Model file for the job. Use its own axes, mm. Face numbers are marked on the shaded views. Round coordinates to 2 decimals unless told otherwise and drop trailing zeros. Order: outer loops, then holes, each group sorted by start corner. A loop starts at its lowest first (then second) coordinate and runs counter-clockwise, first axis right, second up. Notation, with made-up numbers: (31.5, -3.75) - (68.5, -3.75) arc R17 ccw to (68.5, 12.25) - close; hole circle Ø2 at (-17, -30.5). An arc over 180 degrees is marked (long way). Put each result on its own line as item: value. Start each with the question number.
Item 1: Mould opens along X. For the marked faces 1, 2, 3 and 4 say: pulls with the +X half, pulls with the -X half, needs draft (parallel to the pull), parting line crosses it, or undercut.
Item 2: Saw through at A-A on x = 0. List the corners of the cut face in (y, z), plus the area to 3 significant figures.
Item 3: Pin check, flat tips, straight feed: pin 1 Ø1.5 at (x, y) = (6.5, 1.5) entering from +Z; pin 2 Ø3 at (x, y) = (7, 1) entering from -Z; pin 3 Ø1.5 at (x, y) = (3.5, 4) entering from -Z. Stop position of each tip, or through.
Item 4: Saw through at C-C on y = 3.4. List the corners of the cut face in (x, z), plus the area to 3 significant figures.
Item 5: Saw through at D-D on z = 9.25. List the corners of the cut face in (x, y), plus the area to 3 significant figures.
Item 6: Saw through at B-B on z = 0. List the corners of the cut face in (x, y), plus the area to 3 significant figures.
Item 7: Probe probe 1 along X at (y, z) = (1.6, 0); probe 2 along Z at (x, y) = (-1.5, 2.8); probe 3 along Z at (x, y) = (0, 1.55). List the from-to ranges inside material, lowest first.
```python
from build123d import *

# Parameters (mm, degrees)
SKETCH1_R           = 11.25
BOSS_EXTRUDE1_DEPTH = 5.38
SKETCH2_R           = 3
CUT_EXTRUDE1_DEPTH  = 5.38
SKETCH3_W           = 5.871522131
SKETCH3_H           = 2.131460622
BOSS_EXTRUDE2_DEPTH = 5.38


with BuildPart() as part:
    # Sketch1 → Boss-Extrude1 (new body)
    with BuildSketch(Plane(origin=(0, 0, 0), x_dir=(1, 0, 0), z_dir=(0, 1, 0))):
        Circle(SKETCH1_R)
    extrude(amount=BOSS_EXTRUDE1_DEPTH)

    # Sketch2 → Cut-Extrude1 (cut)
    with BuildSketch(Plane(origin=(0, 5.38, 0), x_dir=(1, 0, 0), z_dir=(0, 1, 0))):
        Circle(SKETCH2_R)
    extrude(amount=-CUT_EXTRUDE1_DEPTH, mode=Mode.SUBTRACT)

    # Sketch3 → Boss-Extrude2 (add)
    with BuildSketch(Plane(origin=(0, 5.38, 0), x_dir=(1, 0, 0), z_dir=(0, 1, 0))):
        with Locations((-0.064238934, 1.934269689)):
            Rectangle(SKETCH3_W, SKETCH3_H)
    extrude(amount=-BOSS_EXTRUDE2_DEPTH)


solid = part.part
```
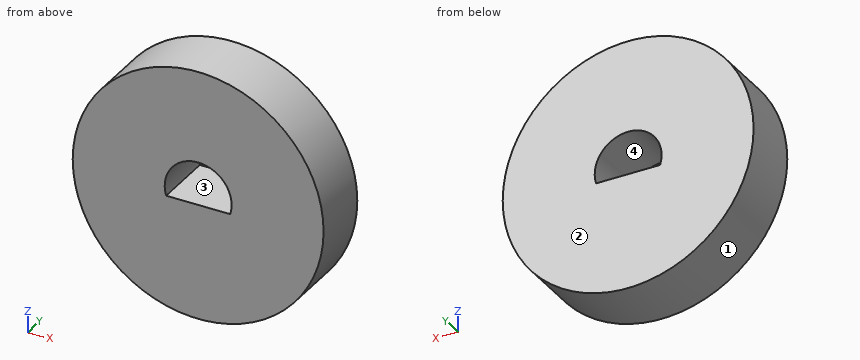
Results found:
1. face 1: parting line crosses it
1. face 2: needs draft
1. face 3: undercut
1. face 4: undercut
2. outline: (0, -11.25) - (5.38, -11.25) - (5.38, -0.87) - (0, -0.87) - close; (0, 3) - (5.38, 3) - (5.38, 11.25) - (0, 11.25) - close
2. area: 100 mm²
3. pin 1: stops at z = 9.67
3. pin 2: stops at z = -9.81
3. pin 3: stops at z = -10.91
4. outline: circle Ø22.5 at (0, 0); hole (-2.87, -0.87) - (2.87, -0.87) arc R3 ccw (long way) to start
4. area: 378 mm²
5. outline: (-6.4, 0) - (6.4, 0) - (6.4, 5.38) - (-6.4, 5.38) - close
5. area: 68.9 mm²
6. outline: (-11.25, 0) - (-3, 0) - (-3, 5.38) - (-11.25, 5.38) - close; (3, 0) - (11.25, 0) - (11.25, 5.38) - (3, 5.38) - close
6. area: 88.8 mm²
7. probe 1: x = -11.25 to -3, 3 to 11.25
7. probe 2: z = -11.15 to -0.87, 2.6 to 11.15
7. probe 3: z = -11.25 to -0.87, 3 to 11.25
